from build123d import *

# Parameters (mm, degrees)
F0_R          = 7.380765
F1_DEPTH      = 57.7
F2_W          = 37.0757319033
F2_H          = 8.3348543849
F3_DEPTH      = 9.1
F3_DEPTH_BACK = 9.4
F4_T1_DEPTH   = 60.2404459759


# Not quite as in the source:
# - a fillet or chamfer that OpenCascade refuses, or shapes differently, is made with other operations: its cross-section is extruded or revolved along the edge and cut away or added


with BuildPart() as f1:
    # F0 (on Front) → F1 (new body)
    with BuildSketch(Plane.XZ):
        Circle(F0_R)
    extrude(amount=F1_DEPTH)

    # F2 (on Top) → F3 (join, two sides)
    with BuildSketch(Plane.XY) as f3_sk:
        with Locations((-0.2874098718, -1.4370438876)):
            Rectangle(F2_W, F2_H)
    extrude(amount=F3_DEPTH)
    extrude(f3_sk.sketch, amount=-F3_DEPTH_BACK)

    # F4: fillet of radius 10.3811183182 on 4 edges, made by hand

    # F4_s2 → F4_t1 (cut)
    with BuildSketch(Plane.XZ.offset(-28.6831791004)):
        with BuildLine():
            ThreePointArc((-18.8252758235, 0.9811183182), (-15.7847166644, -6.3594408409), (-8.4441575053, -9.4))
            Line((-8.4441575053, -9.4), (-18.8252758235, -9.4))
            Line((-18.8252758235, -9.4), (-18.8252758235, 0.9811183182))
        make_face()
        with BuildLine():
            ThreePointArc((-8.4441575053, 9.1), (-15.7847166644, 6.0594408409), (-18.8252758235, -1.2811183182))
            Line((-18.8252758235, -1.2811183182), (-18.8252758235, 9.1))
            Line((-18.8252758235, 9.1), (-8.4441575053, 9.1))
        make_face()
        with BuildLine():
            ThreePointArc((7.8693377616, 9.1), (15.2098969207, 6.0594408409), (18.2504560798, -1.2811183182))
            Line((18.2504560798, -1.2811183182), (18.2504560798, 9.1))
            Line((18.2504560798, 9.1), (7.8693377616, 9.1))
        make_face()
        with BuildLine():
            ThreePointArc((18.2504560798, 0.9811183182), (15.2098969207, -6.3594408409), (7.8693377616, -9.4))
            Line((7.8693377616, -9.4), (18.2504560798, -9.4))
            Line((18.2504560798, -9.4), (18.2504560798, 0.9811183182))
        make_face()
    extrude(amount=F4_T1_DEPTH, mode=Mode.SUBTRACT)


solid = f1.part
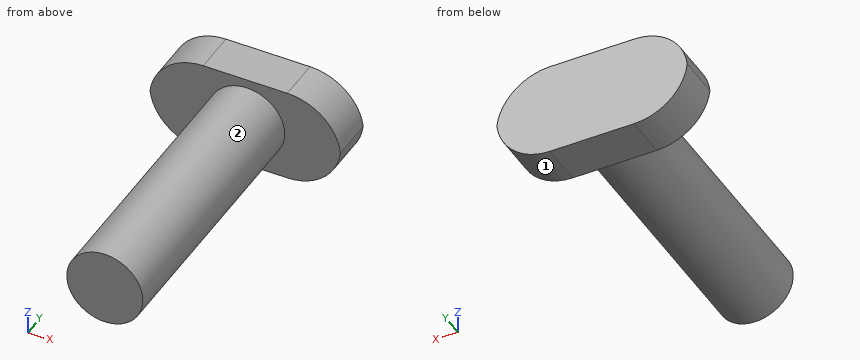
Could you check a few things on this model? Use its own coordinates, in mm. Face numbers are marked on the shaded views. A direction names the side the tool comes from. Give positions to 0.01 mm unless a question says otherwise; leave off trailing zeros. Loops run counter-clockwise (first coordinate to the right, second up) from the corner with the lowest first, then second, coordinate; pieces in that order, holes last. Notation, with made-up numbers: (17.5, 73.25) -> (51.5, 73.25) arc R37 cw to (51.5, 112.25) -> close; hole circle Ø2 at (-27.75, 66). An arc over 180 degrees is marked (long way). Return JSON: item names as keys, results as strings.
Item 1: I'm going to push flat-ended pins straight in: pin 1 (10 mm diameter, centred on y = -40, z = 1.5, fed in from +X); pin 2 (10 mm diameter, centred on y = -20, z = 3.5, fed in from -X); pin 3 (12 mm diameter, centred on x = 0.5, y = -26.5, fed in from -Z). Where does each tip first touch, or does it pass through?
Geometry results:
{"pin 1": "stops at x = 7.38", "pin 2": "stops at x = -7.38", "pin 3": "stops at z = -7.38"}
Item 2: If we section it at B-B on z = -1.25: List the corners of the cut face in (x, y) for me.
Geometry results:
{"outline": "(-18.58, -5.6) -> (-7.27, -5.6) -> (-7.27, -57.7) -> (7.27, -57.7) -> (7.27, -5.6) -> (18.01, -5.6) -> (18.01, 2.73) -> (-18.58, 2.73) -> close"}
Item 3: If we section it at D-D on y = -35.5: List the corners of the cut face in (x, z) for me, plus the area to 3 significant figures.
Geometry results:
{"outline": "circle Ø14.76 at (0, 0)", "area": "171 mm²"}
Item 4: I need wall thicknesses on L1, parallel to Y at x = 10, z = 1.5; L2, parallel to Z at x = -5.5, y = -54.5; L3, parallel to X at y = -55, z = 0. Which ranges of each line are inside material? Lowest first, please. Write a range as from..to.
Geometry results:
{"L1": "y = -5.6..2.73", "L2": "z = -4.92..4.92", "L3": "x = -7.38..7.38"}
Item 5: If we section it at C-C on y = -0.5: List the corners of the cut face in (x, z) for me, plus the area to 3 significant figures.
Geometry results:
{"outline": "(-18.76, -0.15) arc R10.38 ccw to (-8.44, -9.4) -> (7.87, -9.4) arc R10.38 ccw to (18.19, -0.15) arc R10.38 ccw to (7.87, 9.1) -> (-8.44, 9.1) arc R10.38 ccw to start", "area": "593 mm²"}
Item 6: If we section it at A-A on x = 0: List the corners of the cut face in (y, z) for me, plus the area to 3 significant figures.
Geometry results:
{"outline": "(-57.7, -7.38) -> (-5.6, -7.38) -> (-5.6, -9.4) -> (2.73, -9.4) -> (2.73, 9.1) -> (-5.6, 9.1) -> (-5.6, 7.38) -> (-57.7, 7.38) -> close", "area": "923 mm²"}
Item 7: Which directions (+Z, -Z, +X, -X, +Y, -Y) give clear straight access to the entire face, cutting with the end or side of a thin tool? Please do the marked faces 1 and 2.
Geometry results:
{"face 1": "-Z, +X, +Y, -Y", "face 2": "-Y"}
